from build123d import *

# Parameters (mm, degrees)
Y_KSEKLIK_EKSTR_ZYON1_DEPTH = 10
RADYUS1_R                   = 3
RADYUS2_R                   = 50
IZIM2_R                     = 3
KES_EKSTR_ZYON1_DEPTH       = 68
PAH1_SIZE                   = 4


with BuildPart() as part:
    # Çizim1 → Yükseklik-Ekstrüzyon1 (new body)
    with BuildSketch(Plane.XY):
        Polygon((100.428030576, 0), (-19.61722488, 250), (13.66214459, 250), (133.707400046, 0), (13.66214459, -250), (-19.61722488, -250), align=None)
    extrude(amount=Y_KSEKLIK_EKSTR_ZYON1_DEPTH)

    # Radyus1
    radyus1_edges = [part.edges().sort_by_distance(p)[0] for p in [
        (13.66214459, 250, 5),
        (13.66214459, -250, 5),
        (-19.61722488, -250, 5),
        (-19.61722488, 250, 5),
    ]]
    fillet(radyus1_edges, radius=RADYUS1_R)

    # Radyus2
    radyus2_edges = [part.edges().sort_by_distance(p)[0] for p in [
        (133.707400046, 0, 5),
        (100.428030576, 0, 5),
    ]]
    fillet(radyus2_edges, radius=RADYUS2_R)

    # Çizim2 → Kes-Ekstrüzyon1 (cut)
    with BuildSketch(Plane.XY.offset(10)):
        with Locations((32.418057802, -179)):
            Circle(IZIM2_R)
        with Locations((65.910880768, -109)):
            Circle(IZIM2_R)
        with Locations((89.834325744, -59)):
            Circle(IZIM2_R)
        with Locations((65.910880768, 109)):
            Circle(IZIM2_R)
        with Locations((89.834325744, 59)):
            Circle(IZIM2_R)
        with Locations((32.418057802, 179)):
            Circle(IZIM2_R)
    extrude(amount=-KES_EKSTR_ZYON1_DEPTH, mode=Mode.SUBTRACT)

    # Pah1
    pah1_edges = [part.edges().sort_by_distance(p)[0] for p in [
        (29.418057802, -179, 10),
        (62.910880768, -109, 10),
        (86.834325744, -59, 10),
        (62.910880768, 109, 10),
        (86.834325744, 59, 10),
        (29.418057802, 179, 10),
    ]]
    chamfer(pah1_edges, length=PAH1_SIZE)


solid = part.part
The listing builds one solid part. Answer for the finished solid, in the listing's coordinates (mm). A direction names the side the tool comes from. Coordinates: 2 decimals unless noted, no trailing zeros. Order: outer loops, then holes, each group sorted by start corner. A loop starts at its lowest first (then second) coordinate and runs counter-clockwise, first axis right, second up. Notation, with made-up numbers: (33, 72) -> (50, 72) arc R22 ccw to (50, 106) -> close; hole circle Ø1 at (76, 11.25). An arc over 180 degrees is marked (long way). Answer in a Markdown table with one row per item. Add a question column.
Item 1: Find section A-A (z = 2.5). Write down the section's boundary in (x, y), then the cut area to 3 significant figures.
Item 2: Find section B-B (x = 49). Write down the section's boundary in (y, z).
Item 3: Find section C-C (y = -151). Write down the section's boundary in (x, z).
Item 4: Find the intervals of material crossed by L1, parallel to Y at x = 19, z = 7.5; L2, parallel to Y at x = 63, z = 6.75; L3, parallel to Y at x = -10, z = 5.5, in increasing order. Write a range as from..to.
Item 5: Each of these flat-tipped pins is pushed along its axis until it touches: P1, Ø1, axis at y = 170.5, z = 3.5, coming from the +X side; P2, Ø4, axis at y = 77.5, z = 7, coming from the +X side; P3, Ø1, axis at y = -71.5, z = 5.5, coming from the -X side (3 decimals). Where does it stop, or does it pass through?
Item 6: Which of the six approach directions +Z, -Z, +X, -X, +Y, -Y give full straight-line access (tool end or side, diameter ignored) to faces 1 (the face through (35.49, -135.24, 4.93)), 2 (the face through (-2, 250, 5))?
Item 7: Determine the mould class of faces 3 (the face through (93, -17, 10)), 4 (the face through (36.994, 132.104, 4.93)), 5 (the face through (89.142, 55.882, 6.194)) for opening direction X: +X half, -X half, draft (parallel to the pull), parting line (faces both ways), or undercut.
Result set:
| question | item | result |
|---|---|---|
| 1 | outline | (-17.55, -245.7) arc R3 ccw to (-14.85, -250) -> (11.77, -250) arc R3 ccw to (14.48, -248.3) -> (123.31, -21.64) arc R50 ccw to (123.31, 21.64) -> (14.48, 248.3) arc R3 ccw to (11.77, 250) -> (-14.85, 250) arc R3 ccw to (-17.55, 245.7) -> (90.04, 21.64) arc R50 cw to (90.04, -21.64) -> close; hole circle Ø6 at (32.42, -179); hole circle Ø6 at (32.42, 179); hole circle Ø6 at (65.91, -109); hole circle Ø6 at (65.91, 109); hole circle Ø6 at (89.83, -59); hole circle Ø6 at (89.83, 59) |
| 1 | area | 16,500 mm² |
| 2 | outline | (-176.41, 0) -> (-107.1, 0) -> (-107.1, 10) -> (-176.41, 10) -> close; (107.1, 0) -> (176.41, 0) -> (176.41, 10) -> (107.1, 10) -> close |
| 3 | outline | (27.92, 0) -> (61.2, 0) -> (61.2, 10) -> (27.92, 10) -> close |
| 4 | L1 | y = -238.88..-169.58, 169.58..238.88 |
| 4 | L2 | y = -147.25..-111.36, -106.64..-77.95, 77.95..106.64, 111.36..147.25 |
| 4 | L3 | y = -250..-229.97, 229.97..250 |
| 5 | P1 | stops at x = 52.08 |
| 5 | P2 | stops at x = 97.45 |
| 5 | P3 | stops at x = 65.855 |
| 6 | face 1 | +Z, -Z, -X |
| 6 | face 2 | +Z, -Z, +X, -X, +Y |
| 7 | face 3 | draft |
| 7 | face 4 | -X half |
| 7 | face 5 | undercut |
